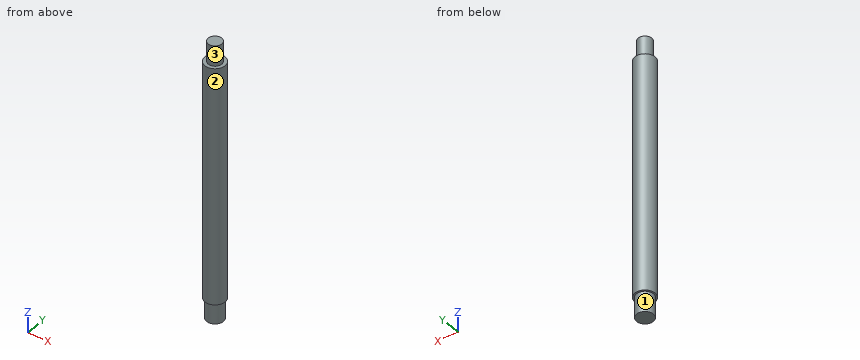
Autodesk Inventor part; units mm, degrees
ref_plane "YZ Plane" through (0, 0, 0) normal (1, 0, 0) x (0, 1, 0)
ref_plane "XZ Plane" through (0, 0, 0) normal (0, 1, 0) x (-1, 0, 0)
ref_plane "XY Plane" through (0, 0, 0) normal (0, 0, 1) x (1, 0, 0)
sketch "Sketch1" plane through (0, 0, 0) normal (0, 0, 1) x (1, 0, 0)
  circle A0 centre (0, 0) radius 6
  dimension "d0" = 12
extrude "Extrusion1" add sketch "Sketch1" along normal blind 152
thread "Thread1"
sketch "Sketch2" plane through (0, 0, 152) normal (0, 0, 1) x (1, 0, 0)
  circle A0 centre (0, 0) radius 6
  circle A1 centre (0, 0) radius 4
  dimension "d5" = 8
extrude "Extrusion2" add sketch "Sketch2" along normal blind 12 contours A1
sketch "Sketch3" plane through (0, 0, 0) normal (0, 0, -1) x (-1, 0, 0)
  circle A0 centre (0, 0) radius 5
  circle A1 centre (0, 0) radius 4
  circle A2 centre (0, 0) radius 6
  dimension "d8" = 10
extrude "Extrusion3" cut sketch "Sketch3" against normal blind 12 contours A2
properties part number "Tornillo de Soporte de Motor" material "Steel"
Part model, mm, in its own coordinate system. Face numbers are marked on the shaded views. A direction names the side the tool comes from. Round coordinates to 2 decimals unless told otherwise and drop trailing zeros. Loops run counter-clockwise (first coordinate to the right, second up) from the corner with the lowest first, then second, coordinate; pieces in that order, holes last. Notation, with made-up numbers: (54, 14) -> (59, 14) arc R5 cw to (59, 21) -> close; hole circle Ø9 at (70.25, 16). An arc over 180 degrees is marked (long way). Use one line per item in the form item = value. Start each with the question number.
Item 1: Tool access for the marked faces 1, 2 and 3: list every direction of +Z, -Z, +X, -X, +Y, -Y with a clear straight run to the whole face (end or side of a thin tool).
Item 2: Drop flat-ended pins along their axis: pin 1 Ø1.5 at (y, z) = (1, 31.5) entering from -X; pin 2 Ø3 at (y, z) = (3.5, 130.5) entering from -X; pin 3 Ø1.5 at (y, z) = (-2.5, 102) entering from +X. Give the stop position or say it passes through.
Item 3: Band-saw the part on C-C (z = 73.5). List the corners of the cut face in (x, y).
Item 4: Drill centre lines: line 1 along X through (y, z) = (4.5, 87); line 2 along Y through (x, z) = (-0.5, 134); line 3 along Z through (x, y) = (3.75, 3). Where is each one in solid material? Low to high.
Item 5: Band-saw the part on A-A (y = 0). List the corners of the cut face in (x, z), plus the area to 3 significant figures.
Data:
q1.face_1 = -Z
q1.face_2 = +Z, -Z
q1.face_3 = +Z
q2.pin_1 = -5.99
q2.pin_2 = -5.66
q2.pin_3 = 5.74
q3.outline = circle Ø12 at (0, 0)
q4.line_1 = -3.97 to 3.97
q4.line_2 = -5.98 to 5.98
q4.line_3 = 0 to 152
q5.outline = (-6, 12) -> (-5, 12) -> (-5, 0) -> (5, 0) -> (5, 12) -> (6, 12) -> (6, 152) -> (4, 152) -> (4, 164) -> (-4, 164) -> (-4, 152) -> (-6, 152) -> close
q5.area = 1,900 mm^2
